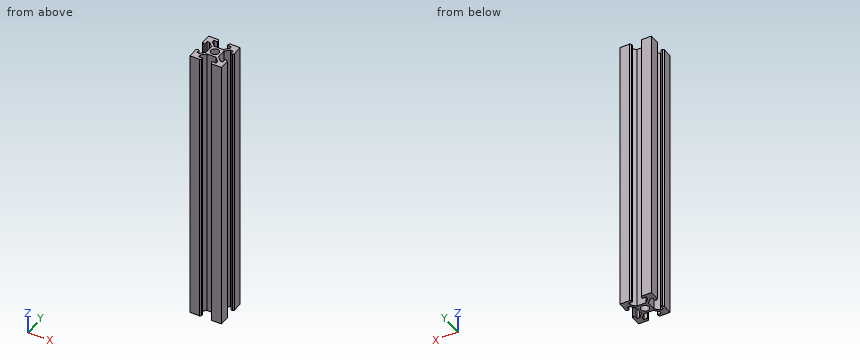
```python
from build123d import *

# Parameters (mm, degrees)
SKETCH1_R           = 2.5
BOSS_EXTRUDE1_DEPTH = 90


with BuildPart() as part:
    # Sketch1 → Boss-Extrude1 (new, symmetric)
    with BuildSketch(Plane.XY):
        Polygon((3.9, -2.839339828), (6.560660172, -5.5), (8.200660172, -5.5), (8.200660172, -3.1), (9.3, -3.1), (10, -3.8), (10, -10), (3.8, -10), (3.1, -9.3), (3.1, -8.200660172), (5.5, -8.200660172), (5.5, -6.560660172), (2.839339828, -3.9), (-2.839339828, -3.9), (-5.5, -6.560660172), (-5.5, -8.200660172), (-3.1, -8.200660172), (-3.1, -9.3), (-3.8, -10), (-10, -10), (-10, -3.8), (-9.3, -3.1), (-8.200660172, -3.1), (-8.200660172, -5.5), (-6.560660172, -5.5), (-3.9, -2.839339828), (-3.9, 2.839339828), (-6.560660172, 5.5), (-8.200660172, 5.5), (-8.200660172, 3.1), (-9.3, 3.1), (-10, 3.8), (-10, 10), (-3.8, 10), (-3.1, 9.3), (-3.1, 8.200660172), (-5.5, 8.200660172), (-5.5, 6.560660172), (-2.839339828, 3.9), (2.839339828, 3.9), (5.5, 6.560660172), (5.5, 8.200660172), (3.1, 8.200660172), (3.1, 9.3), (3.8, 10), (10, 10), (10, 3.8), (9.3, 3.1), (8.200660172, 3.1), (8.200660172, 5.5), (6.560660172, 5.5), (3.9, 2.839339828), align=None)
        with Locations(Location((0, 0, 0), (0, 0, 180))):
            Circle(SKETCH1_R, mode=Mode.SUBTRACT)
    extrude(amount=BOSS_EXTRUDE1_DEPTH, both=True)


solid = part.part
```
Check sheet for the modelled part. Datum: model origin and axes. Units: mm. Give positions to 0.01 mm unless a question says otherwise; leave off trailing zeros. Loops run counter-clockwise (first coordinate to the right, second up) from the corner with the lowest first, then second, coordinate; pieces in that order, holes last. Notation, with made-up numbers: M 26.25,22.25 L 62.25,22.25 A10 cw 62.25,36.25 Z; hole C 79,57 d8. An arc over 180 degrees is marked long. Answer in a Markdown table with one row per item.
1) Depth check by flat-ended pin: pin 1 (4.5 mm diameter, centred on x = 1, z = -32, fed in from +Y); pin 2 (3 mm diameter, centred on x = 1, z = 24.5, fed in from +Y); pin 3 (1.7 mm diameter, centred on x = -1, z = -5, fed in from -Y). Enter the tip coordinate at first touch or a pass-through.
Solutions:
| item | result |
|---|---|
| pin 1 | stops at y = 9.45 |
| pin 2 | stops at y = 3.9 |
| pin 3 | stops at y = -3.9 |
2) Cross-section at A-A (x = 0). Enter the section's corners in (y, z).
Solutions:
| item | result |
|---|---|
| outline | M -3.9,-90 L -2.5,-90 L -2.5,90 L -3.9,90 Z; M 2.5,-90 L 3.9,-90 L 3.9,90 L 2.5,90 Z |
3) Thickness scan on line 1 (Y direction, x = 0, z = 0); line 2 (X direction, y = -3.5, z = -26.5); line 3 (X direction, y = -4.75, z = 57). Record the ranges inside material, lowest first.
Solutions:
| item | result |
|---|---|
| line 1 | y = -3.9 to -2.5, 2.5 to 3.9 |
| line 2 | x = -9.7 to -8.2, -4.56 to 4.56, 8.2 to 9.7 |
| line 3 | x = -10 to -8.2, -5.81 to -3.69, 3.69 to 5.81, 8.2 to 10 |
